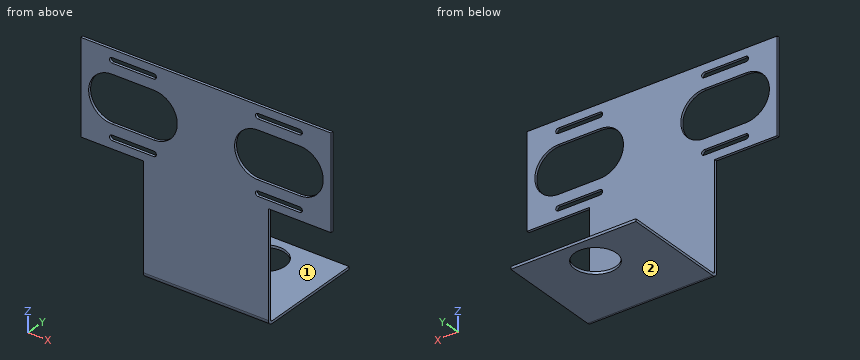
```python
from build123d import *

# Parameters (mm, degrees)
SKETCH1_W              = 304.8
SKETCH1_H              = 114.3
BOSS_EXTRUDE1_DEPTH    = 3.175
CUT_EXTRUDE1_DEPTH     = 163.79423554
SKETCH3_W              = 152.4
SKETCH3_H              = 3.175
BOSS_EXTRUDE2_DEPTH    = 131.445
SKETCH4_W              = 152.4
SKETCH4_H              = 3.175
BOSS_EXTRUDE3_DEPTH    = 133.35
CONVERT_SOLID1_START   = -76.2
CONVERT_SOLID1_DEPTH   = 152.4
CONVERT_SOLID1_2_DEPTH = 152.4
SKETCH5_R              = 25.4
CUT_EXTRUDE2_DEPTH     = 321.888062882


# Read off the part's stored shape, not the designer's step: Convert-Solid1
with BuildPart() as part:
    # Sketch1 → Boss-Extrude1 (new body)
    with BuildSketch(Plane(origin=(0, 0, 0), x_dir=(1, 0, 0), z_dir=(0, 1, 0))):
        Rectangle(SKETCH1_W, SKETCH1_H)
    extrude(amount=BOSS_EXTRUDE1_DEPTH)

    # Sketch2 → Cut-Extrude1 (cut, through all)
    with BuildSketch(Plane(origin=(0, 3.175, 0), x_dir=(1, 0, 0), z_dir=(0, 1, 0))):
        with BuildLine():
            Line((-114.3, -41.275), (-63.5, -41.275))
            ThreePointArc((-63.5, -41.275), (-60.325, -44.45), (-63.5, -47.625))
            Line((-63.5, -47.625), (-114.3, -47.625))
            ThreePointArc((-114.3, -47.625), (-117.475, -44.45), (-114.3, -41.275))
        make_face()
        with BuildLine():
            Line((-114.3, 47.625), (-63.5, 47.625))
            ThreePointArc((-63.5, 47.625), (-60.325, 44.45), (-63.5, 41.275))
            Line((-63.5, 41.275), (-114.3, 41.275))
            ThreePointArc((-114.3, 41.275), (-117.475, 44.45), (-114.3, 47.625))
        make_face()
        with BuildLine():
            Line((-114.3, 28.575), (-63.5, 28.575))
            ThreePointArc((-63.5, 28.575), (-34.925, 0), (-63.5, -28.575))
            Line((-63.5, -28.575), (-114.3, -28.575))
            ThreePointArc((-114.3, -28.575), (-142.875, 0), (-114.3, 28.575))
        make_face()
    cut_extrude1 = extrude(amount=-CUT_EXTRUDE1_DEPTH, mode=Mode.SUBTRACT)

    # Sketch3 → Boss-Extrude2 (add)
    with BuildSketch(Plane.XY.offset(-57.15)):
        with Locations((0, 1.5875)):
            Rectangle(SKETCH3_W, SKETCH3_H)
    extrude(amount=-BOSS_EXTRUDE2_DEPTH)

    # Sketch4 → Boss-Extrude3 (add)
    with BuildSketch(Plane(origin=(0, 0, 0), x_dir=(-1, 0, 0), z_dir=(0, -1, 0))):
        with Locations((0, 190.1825)):
            Rectangle(SKETCH4_W, SKETCH4_H)
    extrude(amount=-BOSS_EXTRUDE3_DEPTH)

    # Convert-Solid1 outline → Convert-Solid1 (cut)
    with BuildSketch(Plane.YZ.offset(CONVERT_SOLID1_START)):
        with BuildLine():
            ThreePointArc((6.35, -191.77), (1.859871939, -189.910128061), (0, -185.42))
            Line((0, -185.42), (0, -191.77))
            Line((0, -191.77), (6.35, -191.77))
        make_face()
    extrude(amount=CONVERT_SOLID1_DEPTH, mode=Mode.SUBTRACT)

    # Convert-Solid1 2 outline → Convert-Solid1 2 (add)
    with BuildSketch(Plane.YZ.offset(CONVERT_SOLID1_START)):
        with BuildLine():
            ThreePointArc((6.35, -188.595), (4.10493597, -187.66506403), (3.175, -185.42))
            Line((3.175, -185.42), (3.175, -188.595))
            Line((3.175, -188.595), (6.35, -188.595))
        make_face()
    extrude(amount=CONVERT_SOLID1_2_DEPTH)

    # Mirror1: Cut-Extrude1 across plane
    add(cut_extrude1.mirror(Plane(origin=(0, 0, 0), x_dir=(0, 0, 1), z_dir=(1, 0, 0))), mode=Mode.SUBTRACT)

    # Sketch5 → Cut-Extrude2 (cut, through all)
    with BuildSketch(Plane(origin=(0, 0, -191.77), x_dir=(-1, 0, 0), z_dir=(0, 0, -1))):
        with Locations((0, 96.8375)):
            Circle(SKETCH5_R)
    extrude(amount=-CUT_EXTRUDE2_DEPTH, mode=Mode.SUBTRACT)


solid = part.part
```
Here's how the part is built. I have some questions about the finished solid (model axes, mm). Face numbers are marked on the shaded views. A direction names the side the tool comes from. Give positions to 0.01 mm unless a question says otherwise; leave off trailing zeros. Write each loop counter-clockwise with the first axis right and the second up, starting at its lowest first coordinate (ties: lowest second). Pieces come first, ordered by that corner, then holes. Notation, with made-up numbers: M 47,19 L 102,19 A18 ccw 102,30 Z; hole C 89,83 d8. An arc over 180 degrees is marked long. Put each result on its own line as item: value. Start each with the question number.
Item 1: If we section it at D-D, the plane x = 17: Write out the boundary of the cut face in (y, z) (3 decimals).
Item 2: If we section it at C-C, the plane y = 105.5: Write out the boundary of the cut face in (x, z) (3 decimals), then the cut area to 3 significant figures.
Item 3: Will these pins go through, and if not, where does the flat tip stop? pin 1 (1 mm diameter, centred on x = -100, y = 2, fed in from -Z); pin 2 (1.5 mm diameter, centred on x = -75.5, z = -109, fed in from +Y) (3 decimals); pin 3 (1.5 mm diameter, centred on x = -59, y = 81.5, fed in from +Z) (3 decimals).
Item 4: If we section it at A-A, the plane x = -45: Write out the boundary of the cut face in (y, z) (3 decimals), then the cut area to 3 significant figures.
Item 5: I need wall thicknesses on L1, parallel to Y at x = 0, z = -189; L2, parallel to Y at x = 8, z = -123 (3 decimals); L3, parallel to Z at x = 61, y = 106.5 (3 decimals). Which ranges of each line are inside material? Lowest first, please. Write a range as from..to.
Item 6: On a 3-axis mill with a long thin cutter (end or side, diameter ignored), from which of +Z, -Z, +X, -X, +Y, -Y can I reach the whole of each face in a straight line? I mean the marked faces 1 and 2. Say none if no direction works.
Item 7: If we section it at B-B, the plane z = 0: Write out the boundary of the cut face in (x, y) (3 decimals).
Values:
1. outline: M 0,-185.42 A6.35 ccw 6.35,-191.77 L 77.965,-191.77 L 77.965,-188.595 L 6.35,-188.595 A3.175 cw 3.175,-185.42 L 3.175,57.15 L 0,57.15 Z; M 115.71,-191.77 L 133.35,-191.77 L 133.35,-188.595 L 115.71,-188.595 Z
2. outline: M -76.2,-191.77 L -23.877,-191.77 L -23.877,-188.595 L -76.2,-188.595 Z; M 23.877,-191.77 L 76.2,-191.77 L 76.2,-188.595 L 23.877,-188.595 Z
2. area: 332 mm²
3. pin 1: z = -57.15
3. pin 2: y = 3.175
3. pin 3: z = -188.595
4. outline: M 0,-185.42 A6.35 ccw 6.35,-191.77 L 133.35,-191.77 L 133.35,-188.595 L 6.35,-188.595 A3.175 cw 3.175,-185.42 L 3.175,-21.778 L 0,-21.778 Z; M 0,21.778 L 3.175,21.778 L 3.175,57.15 L 0,57.15 Z
4. area: 1,060 mm²
5. L1: 1.11..71.44, 122.24..133.35
5. L2: 0..3.175
5. L3: -191.77..-188.595
6. face 1: +Z, +X, -X, +Y
6. face 2: -Z, +X, -X, +Y, -Y
7. outline: M -152.4,0 L -142.875,0 L -142.875,3.175 L -152.4,3.175 Z; M -34.925,0 L 34.925,0 L 34.925,3.175 L -34.925,3.175 Z; M 142.875,0 L 152.4,0 L 152.4,3.175 L 142.875,3.175 Z
